Geometry check sheet. Reference: the model listing, model coordinates, mm. A direction names the side the tool comes from. Round coordinates to 2 decimals unless told otherwise and drop trailing zeros. Order: outer loops, then holes, each group sorted by start corner. A loop starts at its lowest first (then second) coordinate and runs counter-clockwise, first axis right, second up. Notation, with made-up numbers: (-1.5, 34.5) -> (9.5, 34.5) arc R7 cw to (9.5, 40.5) -> close; hole circle Ø1 at (62.5, 48.25). An arc over 180 degrees is marked (long way). Use a Markdown table: item, result. Add a question column.
Item 1: Material ranges on probe 1 along Z at (x, y) = (99.75, -65.5); probe 2 along Y at (x, z) = (106, 7.5); probe 3 along Z at (x, y) = (110, -58.75), recorded low to high. Write a range as [from, to].
Item 2: Set-up check for faces 4 (the conical face through (104.92, -58.08, 5.45)), 5 (the flat face through (106, -61, 0)): record each of +Z, -Z, +X, -X, +Y, -Y from which the full face is reachable in a straight line by a thin tool's end or side.
Item 3: Gauge pin test, flat ends, axial feed: pin 1 Ø8 at (x, y) = (106.3, -64.32) entering from +Z; pin 2 Ø1 at (y, z) = (-69, 3) entering from -X; pin 3 Ø6 at (y, z) = (-60, 6) entering from +X; pin 4 Ø1 at (y, z) = (-59, 8.5) entering from +X. Record the tip position at first contact, or that the pin passes through.
Item 4: Sectioned sample at B-B, the plane z = 8.75. Record the cut outline in (x, y).
Item 5: Mould release check, pull along X, two halves, no side actions. Record for faces 1 (the cylindrical face through (104.95, -58.22, 3.53)), 2 (the cylindrical face through (103.753, -64.209, 5.577)), 3 (the flat face through (104, -66, 11)): pulls with the +X half, pulls with the -X half, needs draft (parallel to the pull), parting line crosses it, or undercut.
Item 6: Sectioned sample at A-A, the plane z = 3. Record the cut outline in (x, y), and give its area (3 significant figures).
from build123d import *

# Parameters (mm, degrees)
F_5_1_5_1_DIAMETER_HOLE1_D     = 5.1
F_5_1_5_1_DIAMETER_HOLE1_DEPTH = 11


with BuildPart() as part:
    # Sketch1 → Revolve1 (revolve)
    with BuildSketch(Plane.XZ.offset(64.320770854)):
        with BuildLine():
            Line((114.770297578, 11), (106.300627664, 11))
            Line((106.300627664, 11), (106.300627664, 0))
            Line((106.300627664, 0), (113.567535888, 0))
            Line((113.567535888, 0), (113.634922783, 0.251491318))
            ThreePointArc((113.634922783, 0.251491318), (113.634922783, 0.510310363), (113.505513261, 0.734454231))
            Line((113.505513261, 0.734454231), (112.550627664, 1.689339828))
            Line((112.550627664, 1.689339828), (112.550627664, 5.310660172))
            Line((112.550627664, 5.310660172), (114.770297578, 7.530330086))
            Line((114.770297578, 7.530330086), (114.770297578, 11))
        make_face()
    revolve(axis=Axis((106.300627664, -64.320770854, 11), (0, 0, -1)))

    # 5.1 _5.1_ Diameter Hole1
    with Locations(Plane(origin=(0, 0, 0), x_dir=(-1, 0, 0), z_dir=(0, 0, -1))):
        with Locations((-106.300627664, -64.320770854)):
            Hole(F_5_1_5_1_DIAMETER_HOLE1_D / 2, depth=F_5_1_5_1_DIAMETER_HOLE1_DEPTH)


solid = part.part
Found:
| question | item | result |
|---|---|---|
| 1 | probe 1 | z = [0, 1.28], [5.72, 11] |
| 1 | probe 2 | y = [-72.75, -66.85], [-61.79, -55.89] |
| 1 | probe 3 | z = [0, 1.25], [5.75, 11] |
| 2 | face 4 | none |
| 2 | face 5 | -Z, +X, -X, +Y, -Y |
| 3 | pin 1 | stops at z = 11 |
| 3 | pin 2 | stops at x = 101.65 |
| 3 | pin 3 | stops at x = 114.59 |
| 3 | pin 4 | stops at x = 113.26 |
| 4 | outline | circle Ø16.94 at (106.3, -64.32); hole circle Ø5.1 at (106.3, -64.32) |
| 5 | face 1 | parting line crosses it |
| 5 | face 2 | undercut |
| 5 | face 3 | needs draft |
| 6 | outline | circle Ø12.5 at (106.3, -64.32); hole circle Ø5.1 at (106.3, -64.32) |
| 6 | area | 102 mm2 |
